Read the model definition and answer for the solid it produces. Units are mm, in the model's axes. A direction names the side the tool comes from. Coordinates: 2 decimals unless noted, no trailing zeros. Write each loop counter-clockwise with the first axis right and the second up, starting at its lowest first coordinate (ties: lowest second). Pieces come first, ordered by that corner, then holes. Notation, with made-up numbers: (-33, -9.75) -> (0, -9.75) arc R20 cw to (0, 28.25) -> close; hole circle Ø3 at (-10, -11). An arc over 180 degrees is marked (long way). Return JSON: item names as keys, results as strings.
Solid Edge part; units mm, degrees
sketch "Sketch1" plane through (0, 0, 6.6) normal (0, 0, 1) x (1, 0, 0)
  line L0 (149.4766, 6.1695) -> (106.2339, 6.1695)
  arc A0 (106.2339, 6.1695) -> (105.2339, 7.1695) centre (106.2339, 7.1695) cw
  line L1 (105.2339, 7.1695) -> (105.2339, 8.0272)
  arc A1 (105.2339, 8.0272) -> (104.2339, 9.0272) centre (104.2339, 8.0272) ccw
  line L2 (104.2339, 9.0272) -> (87.1839, 9.0272)
  arc A2 (87.1839, 9.0272) -> (86.1839, 10.0272) centre (87.1839, 10.0272) cw
  line L3 (86.1839, 10.0272) -> (86.1839, 10.8847)
  arc A3 (86.1839, 10.8847) -> (85.1839, 11.8847) centre (85.1839, 10.8847) ccw
  line L4 (85.1839, 11.8847) -> (48.1339, 11.8847)
  arc A4 (48.1339, 11.8847) -> (47.1339, 10.8847) centre (48.1339, 10.8847) ccw
  line L5 (47.1339, 10.8847) -> (47.1339, 10.0306)
  arc A5 (47.1339, 10.0306) -> (46.1339, 9.0306) centre (46.1339, 10.0306) cw
  line L6 (46.1339, 9.0306) -> (29.0839, 9.0306)
  arc A6 (29.0839, 9.0306) -> (28.0839, 8.0306) centre (29.0839, 8.0306) ccw
  line L7 (28.0839, 8.0306) -> (28.0839, 7.1697)
  arc A7 (28.0839, 7.1697) -> (27.0839, 6.1697) centre (27.0839, 7.1697) cw
  line L8 (27.0839, 6.1697) -> (-9.0161, 6.1697)
  arc A8 (-9.0161, 6.1697) -> (-10.0161, 5.1697) centre (-9.0161, 5.1697) ccw
  line L9 (-10.0161, 5.1697) -> (-10.0161, -111.8903)
  arc A9 (-10.0161, -111.8903) -> (-9.0161, -112.8903) centre (-9.0161, -111.8903) ccw
  line L10 (-9.0161, -112.8903) -> (47.0839, -112.8903)
  arc A10 (47.0839, -112.8903) -> (48.0839, -111.8903) centre (47.0839, -111.8903) ccw
  line L11 (48.0839, -111.8903) -> (48.0839, -111.0328)
  arc A11 (48.0839, -111.0328) -> (49.0839, -110.0328) centre (49.0839, -111.0328) cw
  line L12 (49.0839, -110.0328) -> (66.1339, -110.0328)
  arc A12 (66.1339, -110.0328) -> (67.1339, -109.0328) centre (66.1339, -109.0328) ccw
  line L13 (67.1339, -109.0328) -> (67.1339, -108.1753)
  arc A13 (67.1339, -108.1753) -> (68.1339, -107.1753) centre (68.1339, -108.1753) cw
  line L14 (68.1339, -107.1753) -> (71.8467, -107.1753)
  arc A14 (71.8467, -107.1753) -> (72.3467, -107.3093) centre (71.8467, -108.1753) cw
  line L15 (72.3467, -107.3093) -> (135.2985, -143.6546)
  arc A15 (135.2985, -143.6545) -> (136.6645, -143.2885) centre (135.7985, -142.7885) ccw
  line L16 (136.6646, -143.2885) -> (162.1493, -99.1476)
  arc A16 (162.1493, -99.1476) -> (161.7833, -97.7816) centre (161.2833, -98.6476) ccw
  line L17 (161.7833, -97.7816) -> (150.9766, -91.5423)
  arc A17 (150.9766, -91.5423) -> (150.4766, -90.6763) centre (151.4766, -90.6763) cw
  line L18 (150.4766, -90.6763) -> (150.4766, 5.1695)
  arc A18 (150.4766, 5.1695) -> (149.4766, 6.1695) centre (149.4766, 5.1695) ccw
extrude "Protrusion1" add sketch "Sketch1" along normal blind 3
sketch "Sketch2" plane through (76.1334, -65.9517, 6.6) normal (0, 0, 1) x (1, 0, 0)
  line L0 (39.6416, 62.7117) -> (22.5916, 62.7117)
  arc A0 (21.5916, 63.7117) -> (22.5916, 62.7117) centre (22.5916, 63.7117) ccw
  line L1 (21.5916, 63.7117) -> (21.5916, 64.5692)
  arc A1 (21.5916, 64.5692) -> (20.5916, 65.5692) centre (20.5916, 64.5692) ccw
  line L2 (20.5916, 65.5692) -> (3.5416, 65.5692)
  arc A2 (3.5416, 65.5692) -> (2.5416, 66.5692) centre (3.5416, 66.5692) cw
  line L3 (2.5416, 66.5692) -> (2.5416, 67.4267)
  arc A3 (1.5416, 68.4267) -> (2.5416, 67.4267) centre (1.5416, 67.4267) cw
  line L4 (1.5416, 68.4267) -> (-20.4584, 68.4267)
  arc A4 (-20.4584, 68.4267) -> (-21.4584, 67.4267) centre (-20.4584, 67.4267) ccw
  line L5 (-21.4584, 67.4267) -> (-21.4584, 66.5692)
  arc A5 (-22.4584, 65.5692) -> (-21.4584, 66.5692) centre (-22.4584, 66.5692) ccw
  line L6 (-22.4584, 65.5692) -> (-39.5084, 65.5692)
  arc A6 (-40.5084, 64.5692) -> (-39.5084, 65.5692) centre (-39.5084, 64.5692) cw
  line L7 (-40.5084, 64.5692) -> (-40.5084, 63.7117)
  arc A7 (-41.5084, 62.7117) -> (-40.5084, 63.7117) centre (-41.5084, 63.7117) ccw
  line L8 (-41.5084, 62.7117) -> (-77.6084, 62.7117)
  arc A8 (-77.6084, 62.7117) -> (-78.6084, 61.7117) centre (-77.6084, 61.7117) ccw
  line L9 (-78.6084, 61.7117) -> (-78.6084, -36.4883)
  arc A9 (-77.6084, -37.4883) -> (-78.6084, -36.4883) centre (-77.6084, -36.4883) cw
  line L10 (-77.6084, -37.4883) -> (-36.5584, -37.4883)
  arc A10 (-35.5584, -36.4883) -> (-36.5584, -37.4883) centre (-36.5584, -36.4883) cw
  line L11 (-35.5584, -36.4883) -> (-35.5584, -35.6308)
  arc A11 (-34.5584, -34.6308) -> (-35.5584, -35.6308) centre (-34.5584, -35.6308) ccw
  line L12 (-34.5584, -34.6308) -> (-17.5084, -34.6308)
  arc A12 (-16.5084, -33.6308) -> (-17.5084, -34.6308) centre (-17.5084, -33.6308) cw
  line L13 (-16.5084, -33.6308) -> (-16.5084, -32.7733)
  arc A13 (-15.5084, -31.7733) -> (-16.5084, -32.7733) centre (-15.5084, -32.7733) ccw
  line L14 (-15.5084, -31.7733) -> (-8.5892, -31.7733)
  arc A14 (-8.5892, -31.7733) -> (-8.0892, -31.9072) centre (-8.5892, -32.7733) cw
  line L15 (-8.0892, -31.9073) -> (53.9717, -67.7381)
  arc A15 (53.9717, -67.7381) -> (55.3377, -67.3721) centre (54.4717, -66.8721) ccw
  line L16 (55.3377, -67.3721) -> (74.7757, -33.7045)
  arc A16 (74.7757, -33.7045) -> (74.4097, -32.3384) centre (73.9097, -33.2045) ccw
  line L17 (74.4097, -32.3385) -> (41.1416, -13.1311)
  arc A17 (40.6416, -12.2651) -> (41.1416, -13.1311) centre (41.6416, -12.2651) ccw
  line L18 (40.6416, -12.2651) -> (40.6416, 61.7117)
  arc A18 (39.6416, 62.7117) -> (40.6416, 61.7117) centre (39.6416, 61.7117) cw
extrude "ExtrudedCutout_1" cut sketch "Sketch2" along normal blind 3
sketch "Sketch3" plane through (76.1336, -65.9519, 6.6) normal (0, 0, 1) x (1, 0, 0)
  line L0 (63.6614, 71.1214) -> (63.6614, 39.0756)
  arc A0 (63.6614, 39.0756) -> (62.6614, 38.0756) centre (62.6614, 39.0756) cw
  line L1 (42.7226, 38.0757) -> (62.6614, 38.0756)
  arc A1 (41.7226, 39.0757) -> (42.7226, 38.0757) centre (42.7226, 39.0757) ccw
  line L2 (41.7226, 71.1214) -> (41.7226, 39.0757)
  arc A2 (40.7226, 72.1214) -> (41.7226, 71.1214) centre (40.7226, 71.1214) cw
  line L3 (40.7226, 72.1214) -> (38.7226, 72.1214)
  line L4 (38.7226, 72.1214) -> (38.7226, 76.1215)
  line L5 (66.6614, 76.1215) -> (38.7226, 76.1215)
  line L6 (66.6614, 72.1214) -> (66.6614, 76.1215)
  line L7 (64.6614, 72.1214) -> (66.6614, 72.1214)
  arc A3 (63.6614, 71.1214) -> (64.6614, 72.1214) centre (64.6614, 71.1214) cw
  line L8 (60.3851, 24.4582) -> (60.3851, 15.3706)
  arc A4 (60.3851, 15.3706) -> (61.3851, 14.3706) centre (61.3851, 15.3706) ccw
  line L9 (73.343, 14.3706) -> (61.3851, 14.3706)
  arc A5 (73.343, 14.3706) -> (74.343, 13.3706) centre (73.343, 13.3706) cw
  line L10 (74.343, 13.3706) -> (74.343, 11.3706)
  line L11 (74.343, 11.3706) -> (78.343, 11.3706)
  line L12 (78.343, 11.3706) -> (78.343, 28.4581)
  line L13 (74.343, 28.4581) -> (78.343, 28.4581)
  line L14 (74.343, 26.4581) -> (74.343, 28.4581)
  arc A6 (74.343, 26.4581) -> (73.343, 25.4582) centre (73.343, 26.4582) cw
  line L15 (73.343, 25.4582) -> (61.3851, 25.4582)
  arc A7 (61.3851, 25.4582) -> (60.3851, 24.4582) centre (61.3851, 24.4582) ccw
extrude "ExtrudedCutout_2" cut sketch "Sketch3" along normal blind 3
properties material "ABS Plastic, high impact"
1. The part is cut by section B-B (x = 23.5). Determine the outline of the cut face in (y, z), then the cut area to 3 significant figures.
Taken from the geometry:
{"outline": "(-112.89, 6.6) -> (-103.44, 6.6) -> (-103.44, 9.6) -> (-112.89, 9.6) -> close; (-3.24, 6.6) -> (6.17, 6.6) -> (6.17, 9.6) -> (-3.24, 9.6) -> close", "area": "56.6 mm2"}
2. For a pull along X with two mould halves and no side action, classify faces 1 (the face through (141.05, -116.73, 8.08)), 2 (the face through (156.46, -94.71, 8.08)), 3 (the face through (120, -54, 6.6)) as +X half, -X half, draft (parallel to the pull), parting line (faces both ways), or undercut.
Taken from the geometry:
{"face 1": "undercut", "face 2": "+X half", "face 3": "draft"}
3. A tool of negligible diameter and unlimited length cuts with its end or side. For faces 4 (the face through (98.6, -115.5, 8.1)), 5 (the face through (149.229, -121.527, 8.079)), from which of +Z, -Z, +X, -X, +Y, -Y can it reach the whole face along a straight path? Write none if from no direction.
Taken from the geometry:
{"face 4": "+Z, -Z", "face 5": "+Z, -Z, +X, -Y"}
4. The part is cut by section A-A (y = -24). Determine the outline of the cut face in (x, z) (3 decimals).
Taken from the geometry:
{"outline": "(-10.016, 6.6) -> (-2.475, 6.6) -> (-2.475, 9.6) -> (-10.016, 9.6) -> close; (116.775, 6.6) -> (117.856, 6.6) -> (117.856, 9.6) -> (116.775, 9.6) -> close; (139.795, 6.6) -> (150.477, 6.6) -> (150.477, 9.6) -> (139.795, 9.6) -> close"}
5. The part is cut by section C-C (y = -123.5). Determine the outline of the cut face in (x, z), then the cut area to 3 significant figures.
Taken from the geometry:
{"outline": "(100.39, 6.6) -> (112.46, 6.6) -> (112.46, 9.6) -> (100.39, 9.6) -> close; (137.14, 6.6) -> (148.09, 6.6) -> (148.09, 9.6) -> (137.14, 9.6) -> close", "area": "69.0 mm2"}
6. Flat-ended cylindrical pins translate along their axes: pin 1 Ø1 at (y, z) = (-104, 8) entering from +X; pin 2 Ø0.9 at (y, z) = (-108.5, 8.5) entering from +X; pin 3 Ø1 at (x, z) = (63, 7.5) entering from -Y; pin 4 Ø5 at (x, y) = (120.5, -10.5) entering from -Z. Find the tip coordinate at first contact, or state that the pin passes through.
Taken from the geometry:
{"pin 1": "stops at x = 159.64", "pin 2": "stops at x = 157.01", "pin 3": "stops at y = -110.03", "pin 4": "passes through"}
7. Consider L1, parallel to Y at x = 24, z = 8.85; L2, parallel to X at y = -78.5, z = 9.25 (3 decimals); L3, parallel to Y at x = 63, z = 9.5 (3 decimals). Determine where each line is inside the solid, lowest interval first.
Taken from the geometry:
{"L1": "y = -112.89 to -103.44, -3.24 to 6.17", "L2": "x = -10.016 to -2.475, 116.816 to 150.477", "L3": "y = -110.033 to -97.725, 2.475 to 11.885"}
